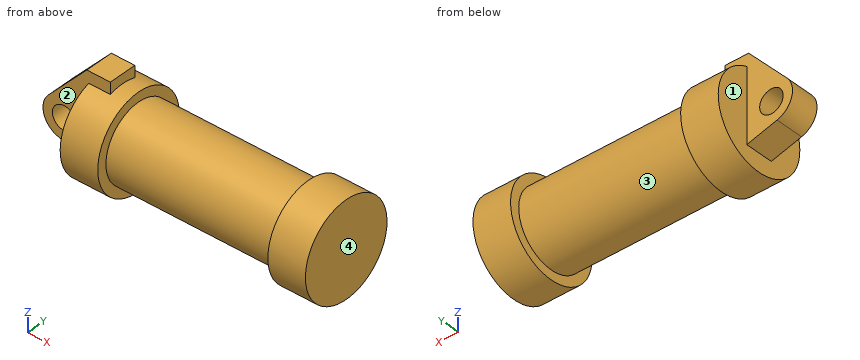
from build123d import *

# Parameters (mm, degrees)
F0_W     = 5.842
F0_H     = 12.7
F0_R     = 3.175
F2_DEPTH = 3.81


# Not quite as in the source:
# - a feature of the source that left no trace in its solid (it failed there, or was rolled back) is left out


with BuildPart() as f1:
    # F0 (on Front) → F1 (revolve)
    with BuildSketch(Plane.XZ):
        Polygon((5.842, 12.7), (5.842, 0), (66.294, 0), (66.294, 12.7), (56.134, 12.7), (56.134, 10.16), (10.16, 10.16), (10.16, 12.7), align=None)
        with Locations((2.921, 6.35)):
            Rectangle(F0_W, F0_H)
    revolve(axis=Axis((33.147, 0, 0), (-1, 0, 0)))

    # F0 (on Front) → F2 (join, symmetric)
    with BuildSketch(Plane.XZ):
        with BuildLine():
            Line((-0.9398, 0), (0, 0))
            Line((0, 0), (0, 12.7))
            Line((0, 12.7), (5.842, 12.7))
            Line((5.842, 12.7), (5.842, 15.24))
            Line((5.842, 15.24), (-0.508, 15.24))
            Line((-0.508, 15.24), (-10.8806298187, 3.8475430269))
            ThreePointArc((-10.8806298187, 3.8475430269), (-4.5919612295, 5.3297205562), (-0.9398, 0))
        make_face()
        with BuildLine():
            ThreePointArc((-8.1826630726, -5.5069827884), (-3.1957909266, -4.5493385486), (-0.9398, 0))
            ThreePointArc((-0.9398, 0), (-4.5919612295, 5.3297205562), (-10.8806298187, 3.8475430269))
            ThreePointArc((-10.8806298187, 3.8475430269), (-12.1459778134, -1.5837270034), (-8.1826630726, -5.5069827884))
        make_face()
        with Locations((-6.6548, 0)):
            Circle(F0_R, mode=Mode.SUBTRACT)
        with BuildLine():
            Line((0, -7.7771894014), (0, 0))
            Line((0, 0), (-0.9398, 0))
            ThreePointArc((-0.9398, 0), (-3.1957909266, -4.5493385486), (-8.1826630726, -5.5069827884))
            Line((-8.1826630726, -5.5069827884), (0, -7.7771894014))
        make_face()
        with Locations((2.921, 6.35)):
            Rectangle(F0_W, F0_H)
        Polygon((5.842, 0), (0, 0), (0, -7.7771894014), (5.842, -9.398), align=None)
    extrude(amount=F2_DEPTH, both=True)


solid = f1.part
Geometry check sheet. Reference: the model listing, model coordinates, mm. Face numbers are marked on the shaded views. Give positions to 0.01 mm unless a question says otherwise; leave off trailing zeros. Loops run counter-clockwise (first coordinate to the right, second up) from the corner with the lowest first, then second, coordinate; pieces in that order, holes last. Notation, with made-up numbers: M 34.5,21 L 57.5,21 A6 ccw 57.5,30 Z; hole C 32.5,49 d7. An arc over 180 degrees is marked long. Write each question's results on one line, items separated by ' | '.
1) Section check B-B, the plane z = 0. Record the boundary of the cut face in (x, y), plus the area to 3 significant figures.
Answers follow:
outline: M -12.37,-3.81 L -9.83,-3.81 L -9.83,3.81 L -12.37,3.81 Z; M -3.48,-3.81 L 0,-3.81 L 0,-12.7 L 10.16,-12.7 L 10.16,-10.16 L 56.13,-10.16 L 56.13,-12.7 L 66.29,-12.7 L 66.29,12.7 L 56.13,12.7 L 56.13,10.16 L 10.16,10.16 L 10.16,12.7 L 0,12.7 L 0,3.81 L -3.48,3.81 Z | area: 1,500 mm2
2) Section check C-C, the plane x = 5. Record the boundary of the cut face in (y, z), plus the area to 3 significant figures.
Answers follow:
outline: M -3.81,12.12 A12.7 ccw long 3.81,12.12 L 3.81,15.24 L -3.81,15.24 Z | area: 528 mm2
3) Gauge pin test, flat ends, axial feed: pin 1 (3 mm diameter, centred on x = 45, y = -7.5, fed in from +Z); pin 2 (1 mm diameter, centred on x = 21, z = 3, fed in from +Y); pin 3 (5.5 mm diameter, centred on x = -5, z = 4, fed in from -Y); pin 4 (7.5 mm diameter, centred on y = 6, z = 0, fed in from -X). Record the tip position at first contact, or that the pin passes through.
Answers follow:
pin 1: z = 8.2 | pin 2: y = 9.85 | pin 3: y = -3.81 | pin 4: x = -12.37
4) Release check for a two-part mould opening along X. For the marked faces 1, 2, 3 and 4 record: +X half, -X half, draft (parallel to the pull), parting line (faces both ways), or undercut.
Answers follow:
face 1: -X half | face 2: draft | face 3: undercut | face 4: +X half
5) Section check D-D, the plane y = 6.75. Record the boundary of the cut face in (x, z), plus the area to 3 significant figures.
Answers follow:
outline: M 0,-10.76 L 10.16,-10.76 L 10.16,-7.59 L 56.13,-7.59 L 56.13,-10.76 L 66.29,-10.76 L 66.29,10.76 L 56.13,10.76 L 56.13,7.59 L 10.16,7.59 L 10.16,10.76 L 0,10.76 Z | area: 1,140 mm2
6) Thickness scan on line 1 (X direction, y = -7.5, z = -9.5); line 2 (Y direction, x = -2.5, z = 6.5); line 3 (X direction, y = 1.75, z = -2). Record the ranges inside material, lowest first.
Answers follow:
line 1: 0 to 10.16, 56.13 to 66.29 | line 2: -3.81 to 3.81 | line 3: -12.01 to -9.12, -4.19 to 66.29
7) Section check A-A, the plane y = 0. Record the boundary of the cut face in (x, z) (3 decimals).
Answers follow:
outline: M -10.881,3.848 A5.715 ccw -8.183,-5.507 L 0,-7.777 L 0,-12.7 L 10.16,-12.7 L 10.16,-10.16 L 56.134,-10.16 L 56.134,-12.7 L 66.294,-12.7 L 66.294,12.7 L 56.134,12.7 L 56.134,10.16 L 10.16,10.16 L 10.16,12.7 L 5.842,12.7 L 5.842,15.24 L -0.508,15.24 Z; hole C -6.655,0 d6.35
